For this review, take the finished solid that the model builds, in its own axes (mm). Give positions to 0.01 mm unless a question says otherwise; leave off trailing zeros. Order: outer loops, then holes, each group sorted by start corner. A loop starts at its lowest first (then second) coordinate and runs counter-clockwise, first axis right, second up.
Item 1: Consider section A-A (y = 0). Give the boundary of the cut face in (x, z), plus the area to 3 significant figures.
Item 2: Consider section C-C (x = -1.35). Give the boundary of the cut face in (y, z), plus the area to 3 significant figures.
Item 3: The part is to be moulded in two halves that separate along X. For faces 1 (the flat face through (2.8, -5, -14)), 2 (the flat face through (-2.8, -5, -14)), 3 (the flat face through (0.04, -1.1, 14.76)), 4 (the flat face through (-0.04, 1.1, 14.76)), say which applies: released by +X, released by -X, zero draft, split by the parting line, or undercut.
Item 4: For P1, Ø3, axis at x = -2, y = 11.5, coming from the -Z side, flat-tipped, find the tip position at first contact; note if it passes through.
Item 5: Consider section B-B (x = 1.55). Give the boundary of the cut face in (y, z), plus the area to 3 significant figures.
Item 6: For probe 1 along Y at (x, z) = (-0.35, 0); probe 2 along Z at (x, y) = (-1.1, 5); probe 3 along Z at (x, y) = (0.2, 0), list the stretches that pass through material, from the lowest coordinate up.
```python
from build123d import *

# Parameters (mm, degrees)
SKETCH_1_W          = 5.6
SKETCH_1_H          = 2
CUT_EXTRUDE_1_DEPTH = 17
FILLET_1_R          = 0.4


with BuildPart() as part:
    # Эскиз1 → Повернуть1 (revolve)
    with BuildSketch(Plane.XY):
        with Locations((0, 15)):
            Rectangle(SKETCH_1_W, SKETCH_1_H)
    revolve(axis=Axis((0, 0, 0), (1, 0, 0)))

    # Эскиз2 → Вырез-Вытянуть1 (cut, through all)
    with BuildSketch(Plane.XY):
        Polygon((2.8, -3.860660172), (-3.860660172, 2.8), (-2.8, 3.860660172), (3.860660172, -2.8), align=None)
    extrude(amount=CUT_EXTRUDE_1_DEPTH, mode=Mode.SUBTRACT)

    # Скругление1
    fillet_1_edges = [part.edges().sort_by_distance(p)[0] for p in [
        (-2.8, -11.912796423, -10.681071172),
        (2.8, -9.854680037, -12.604970503),
        (-2.8, -10.496446008, -9.264157879),
        (2.8, -8.424688647, -11.181440927),
    ]]
    fillet(fillet_1_edges, radius=FILLET_1_R)


solid = part.part
```
Resolved:
1. outline: (-2.8, -15.6) arc R0.4 ccw to (-2.4, -16) - (2.4, -16) arc R0.4 ccw to (2.8, -15.6) - (2.8, -14.4) arc R0.4 ccw to (2.4, -14) - (-2.4, -14) arc R0.4 ccw to (-2.8, -14.4) - close; (-2.8, 14.4) arc R0.4 ccw to (-2.4, 14) - (-1.06, 14) - (-1.06, 16) - (-2.4, 16) arc R0.4 ccw to (-2.8, 15.6) - close; (1.06, 14) - (2.4, 14) arc R0.4 ccw to (2.8, 14.4) - (2.8, 15.6) arc R0.4 ccw to (2.4, 16) - (1.06, 16) - close
1. area: 17.9 mm2
2. outline: (0.29, 14) - (0.29, 16) arc R16 ccw (long way) to (2.41, 15.82) - (2.41, 13.79) arc R14 cw (long way) to start
2. area: 184 mm2
3. face 1: released by +X
3. face 2: released by -X
3. face 3: undercut
3. face 4: undercut
4. P1: stops at z = -12.49
5. outline: (-2.61, 13.75) - (-2.61, 15.79) arc R16 ccw (long way) to (-0.49, 15.99) - (-0.49, 13.99) arc R14 cw (long way) to start
5. area: 184 mm2
6. probe 1: y = -16 to -14, 14 to 16
6. probe 2: z = -15.2 to -13.08, 13.08 to 15.2
6. probe 3: z = -16 to -14
